Check sheet for the modelled part. Datum: model origin and axes. Units: mm. Face numbers are marked on the shaded views. Round coordinates to 2 decimals unless told otherwise and drop trailing zeros. Write each loop counter-clockwise with the first axis right and the second up, starting at its lowest first coordinate (ties: lowest second). Pieces come first, ordered by that corner, then holes. Notation, with made-up numbers: (-37, -11) -> (-30, -11) arc R31 cw to (-30, 21) -> close; hole circle Ø7 at (37, 56). An arc over 180 degrees is marked (long way). One line per item, written item: value. Start each with the question number.
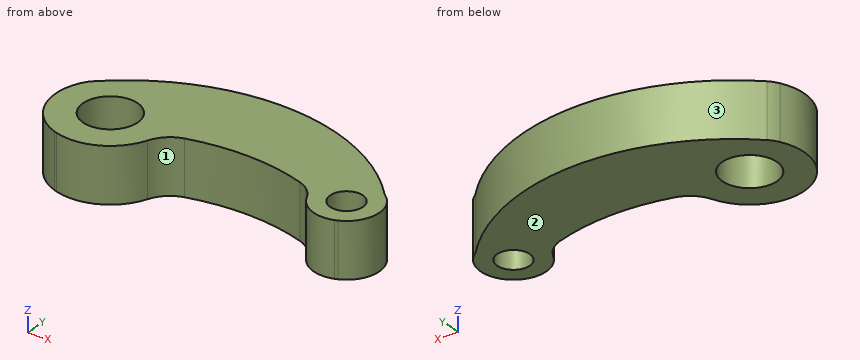
```python
from build123d import *

# Parameters (mm, degrees)
F0_R     = 12.5
F0_R_2   = 7.5
F1_DEPTH = 25


with BuildPart() as f1:
    # F0 (on Top) → F1 (new body)
    with BuildSketch(Plane.XY):
        with BuildLine():
            ThreePointArc((-79.5439328464, 105.0329916801), (-81.1903795815, 103.1025246973), (-82.4879081903, 100.9221785934))
            ThreePointArc((-82.4879081903, 100.9221785934), (-83.0645935002, 80.3550776743), (-68.0186809889, 66.3208793407))
            ThreePointArc((-68.0186809889, 66.3208793407), (-67.296498316, 67.0535704822), (-66.5664236158, 67.7783980852))
            ThreePointArc((-66.5664236158, 67.7783980852), (-66.6515105536, 66.8502006193), (-66.7226044544, 65.9208266473))
            ThreePointArc((-66.7226044544, 65.9208266473), (-48.415623534, 67.8459434438), (-36.3892582797, 81.7821611469))
            ThreePointArc((-36.3892582797, 81.7821611469), (-32.5421815269, 87.7377169865), (-26.3895907314, 91.2611061791))
            ThreePointArc((-26.3895907314, 91.2611061791), (0.5889591855, 94.9981743355), (27.5190997352, 90.926889036))
            ThreePointArc((27.5190997352, 90.926889036), (32.8402812409, 88.0400857367), (36.5869893622, 83.2850059099))
            ThreePointArc((36.5869893622, 83.2850059099), (44.4886785219, 76.049181545), (55.2022156282, 75.9309931922))
            ThreePointArc((55.2022156282, 75.9309931922), (54.9958309784, 76.7755396556), (54.7775992327, 77.6171026405))
            ThreePointArc((54.7775992327, 77.6171026405), (55.5970680513, 77.0322401602), (56.4102927908, 76.4387262274))
            ThreePointArc((56.4102927908, 76.4387262274), (64.1063809456, 84.8999983709), (63.6005239797, 96.3265905096))
            ThreePointArc((63.6005239797, 96.3265905096), (61.3548283708, 99.0601930849), (59.0101731037, 101.7094049462))
            ThreePointArc((59.0101731037, 101.7094049462), (58.1789475446, 102.4000301137), (57.3401107186, 103.0813903939))
            ThreePointArc((57.3401107186, 103.0813903939), (57.8001000902, 102.8124329689), (58.2502464871, 102.5273074881))
            ThreePointArc((58.2502464871, 102.5273074881), (-10.1185209211, 132.8339833721), (-79.5439328464, 105.0329916801))
        make_face()
        with Locations((-60, 90)):
            Circle(F0_R, mode=Mode.SUBTRACT)
        with Locations((50, 90)):
            Circle(F0_R_2, mode=Mode.SUBTRACT)
        with BuildLine():
            ThreePointArc((-66.5664236158, 67.7783980852), (-67.296498316, 67.0535704822), (-68.0186809889, 66.3208793407))
            ThreePointArc((-68.0186809889, 66.3208793407), (-67.3733564047, 66.1120613001), (-66.7226044544, 65.9208266473))
            ThreePointArc((-66.7226044544, 65.9208266473), (-66.6515105536, 66.8502006193), (-66.5664236158, 67.7783980852))
        make_face()
        with BuildLine():
            ThreePointArc((59.0101731037, 101.7094049462), (58.6313959204, 102.1194582653), (58.2502464871, 102.5273074881))
            ThreePointArc((58.2502464871, 102.5273074881), (57.8001000902, 102.8124329689), (57.3401107186, 103.0813903939))
            ThreePointArc((57.3401107186, 103.0813903939), (58.1789475446, 102.4000301137), (59.0101731037, 101.7094049462))
        make_face()
        with BuildLine():
            ThreePointArc((61.7653971487, 99.3045918735), (60.1367140397, 101.056537816), (58.2502464871, 102.5273074881))
            ThreePointArc((58.2502464871, 102.5273074881), (58.6313959204, 102.1194582653), (59.0101731037, 101.7094049462))
            ThreePointArc((59.0101731037, 101.7094049462), (60.3990725447, 100.5199305447), (61.7653971487, 99.3045918736))
        make_face()
        with BuildLine():
            ThreePointArc((63.6005239797, 96.3265905096), (62.7700670204, 97.8692685998), (61.7653971487, 99.3045918735))
            ThreePointArc((61.7653971487, 99.3045918736), (60.3990725447, 100.5199305447), (59.0101731037, 101.7094049462))
            ThreePointArc((59.0101731037, 101.7094049462), (61.3548283708, 99.0601930849), (63.6005239797, 96.3265905096))
        make_face()
        with BuildLine():
            ThreePointArc((55.2022156282, 75.9309931922), (55.8118014552, 76.1716608428), (56.4102927908, 76.4387262274))
            ThreePointArc((56.4102927908, 76.4387262274), (55.5970680513, 77.0322401602), (54.7775992327, 77.6171026405))
            ThreePointArc((54.7775992327, 77.6171026405), (54.9958309784, 76.7755396556), (55.2022156282, 75.9309931922))
        make_face()
    extrude(amount=F1_DEPTH)


solid = f1.part
```
1. Cross-section at D-D (y = 116). Record the cut outline in (x, z).
2. Cross-section at C-C (x = 50). Record the cut outline in (y, z).
3. Depth check by flat-ended pin: pin 1 Ø2 at (x, z) = (2.5, 5) entering from -Y; pin 2 Ø4 at (y, z) = (109, 4.5) entering from -X; pin 3 Ø3 at (y, z) = (113, 5) entering from -X; pin 4 Ø3 at (x, y) = (48, 116) entering from -Z. Enter the tip coordinate at first touch or a pass-through.
4. Material ranges on probe 1 along X at (y, z) = (100.5, 23.25); probe 2 along X at (y, z) = (100, 18); probe 3 along Y at (x, z) = (-60, 16), recorded low to high.
5. Release check for a two-part mould opening along X. For the marked faces 1, 2 and 3 record: +X half, -X half, draft (parallel to the pull), parting line (faces both ways), or undercut.
6. Cross-section at B-B (x = -60). Record the cut outline in (y, z).
7. Cross-section at A-A (z = 21.25). Record the cut outline in (x, y) (3 decimals).
Working result:
1. outline: (-66.27, 0) -> (42.53, 0) -> (42.53, 25) -> (-66.27, 25) -> close
2. outline: (75, 0) -> (82.5, 0) -> (82.5, 25) -> (75, 25) -> close; (97.5, 0) -> (110.33, 0) -> (110.33, 25) -> (97.5, 25) -> close
3. pin 1: stops at y = 94.94
3. pin 2: stops at x = -77.5
3. pin 3: stops at x = -72.31
3. pin 4: passes through
4. probe 1: x = -82.69 to -66.78, -53.22 to 60.71
4. probe 2: x = -82.91 to -67.5, -52.5 to 61.18
4. probe 3: y = 65 to 77.5, 102.5 to 119.95
5. face 1: undercut
5. face 2: draft
5. face 3: parting line
6. outline: (65, 0) -> (77.5, 0) -> (77.5, 25) -> (65, 25) -> close; (102.5, 0) -> (119.95, 0) -> (119.95, 25) -> (102.5, 25) -> close
7. outline: (-82.488, 100.922) arc R25 ccw (long way) to (-36.389, 81.782) arc R15 cw to (-26.39, 91.261) arc R95 cw to (27.519, 90.927) arc R15 cw to (36.587, 83.285) arc R15 ccw (long way) to (58.25, 102.527) arc R96.233 ccw to (-79.544, 105.033) arc R15 ccw to start; hole circle Ø25 at (-60, 90); hole circle Ø15 at (50, 90)
